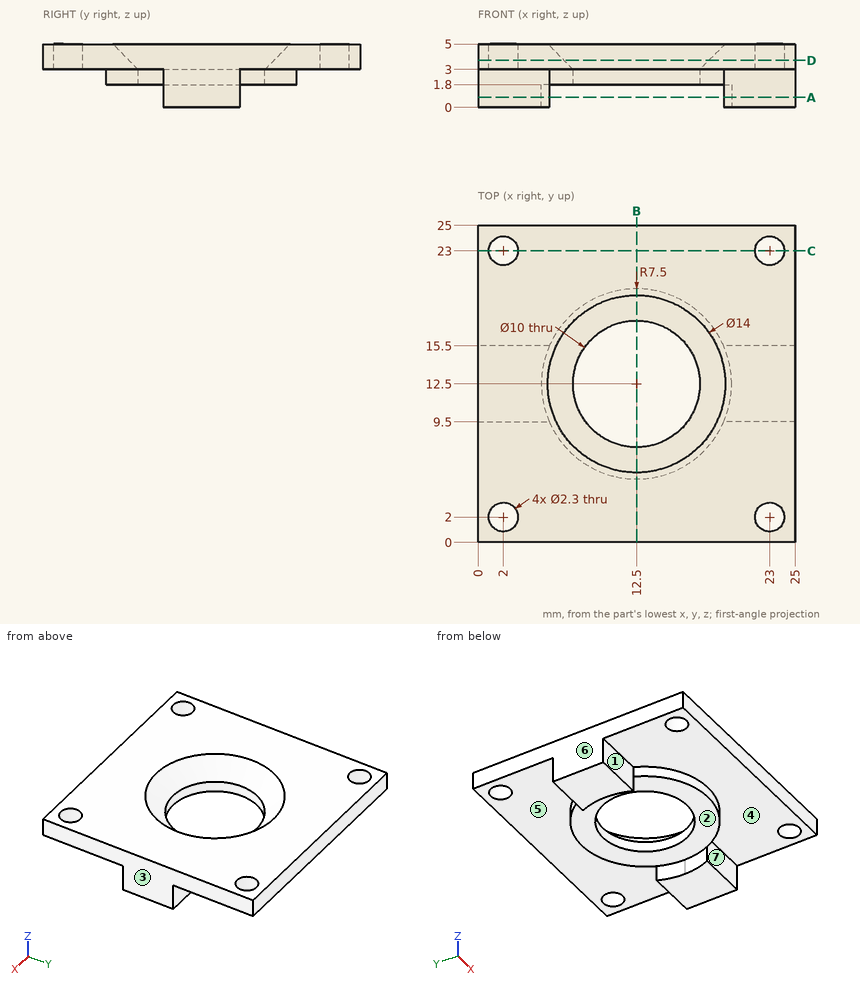
The figure shows three views and two pictorial views of one solid part (mm, origin at its lowest corner). Answer the questions. A direction names the side the tool comes from. Coordinates: 2 decimals unless noted, no trailing zeros. Order: outer loops, then holes, each group sorted by start corner. A loop starts at its lowest first (then second) coordinate and runs counter-clockwise, first axis right, second up. Notation, with made-up numbers: (-30, -24) - (25, -24) arc R14 ccw to (25, -10) - close; hole circle Ø11 at (-5, 38.5). An arc over 180 degrees is marked (long way). Answer as a JSON object with one key per item and string values.
1. Each of these flat-tipped pins is pushed along its axis until it touches: P1, Ø7.5, axis at x = 10, y = 9.5, coming from the -Z side; P2, Ø2.5, axis at x = 23, y = 23, coming from the +Z side; P3, Ø1.5, axis at x = 1.5, z = 1.5, coming from the -Y side; P4, Ø2, axis at x = 19.5, y = 5, coming from the -Z side. Where does it stop, or does it pass through?
Output values:
{"P1": "stops at z = 1.8", "P2": "stops at z = 5", "P3": "stops at y = 9.5", "P4": "stops at z = 3"}
2. Find section B-B on x = 12.5. Determine the outline of the cut face in (y, z).
Output values:
{"outline": "(0, 3) - (5, 3) - (5, 1.8) - (7.5, 1.8) - (7.5, 3) - (5.5, 5) - (0, 5) - close; (17.5, 1.8) - (20, 1.8) - (20, 3) - (25, 3) - (25, 5) - (19.5, 5) - (17.5, 3) - close"}
3. Find section D-D on z = 3.7. Determine the outline of the cut face in (x, y).
Output values:
{"outline": "(0, 0) - (25, 0) - (25, 25) - (0, 25) - close; hole circle Ø2.3 at (2, 2); hole circle Ø2.3 at (2, 23); hole circle Ø11.4 at (12.5, 12.5); hole circle Ø2.3 at (23, 2); hole circle Ø2.3 at (23, 23)"}
4. Find section C-C on y = 23. Determine the outline of the cut face in (x, z).
Output values:
{"outline": "(0, 3) - (0.85, 3) - (0.85, 5) - (0, 5) - close; (3.15, 3) - (21.85, 3) - (21.85, 5) - (3.15, 5) - close; (24.15, 3) - (25, 3) - (25, 5) - (24.15, 5) - close"}
5. Find section A-A on z = 0.8. Determine the outline of the cut face in (x, y).
Output values:
{"outline": "(0, 9.5) - (5.63, 9.5) arc R7.5 cw to (5.63, 15.5) - (0, 15.5) - close; (19.37, 9.5) - (25, 9.5) - (25, 15.5) - (19.37, 15.5) arc R7.5 cw to (20, 12.5) arc R7.5 cw to start"}
6. Consider line 1 (X direction, y = 2, z = 4.1); line 2 (X direction, y = 12.5, z = 2.35). Determine where each line is inside the solid, lowest interval first.
Output values:
{"line 1": "x = 0 to 0.85, 3.15 to 21.85, 24.15 to 25", "line 2": "x = 0 to 7.5, 17.5 to 25"}
7. The mould has two halves that part along X. Classify the marked faces 1, 2 and 3: +X half, -X half, draft (parallel to the pull), parting line (faces both ways), or undercut.
Output values:
{"face 1": "draft", "face 2": "undercut", "face 3": "+X half"}
8. A tool of negligible diameter and unlimited length cuts with its end or side. For the marked faces 4, 5, 6 and 7, from which of +Z, -Z, +X, -X, +Y, -Y can it reach the whole face along a straight path? Write none if from no direction.
Output values:
{"face 4": "-Z, -Y", "face 5": "-Z, +Y", "face 6": "+Z, -Z, -X, +Y, -Y", "face 7": "-Z, +X, -Y"}
